from build123d import *

# Parameters (mm, degrees)
BOX_W           = 11
BOX_H           = 19
BOX_DEPTH       = 8
CHAMFER_SIZE    = 3
CHAMFER002_SIZE = 3


with BuildPart() as part:
    # Box → Box (new body)
    with BuildSketch(Plane.XY):
        with Locations((5.5, 9.5)):
            Rectangle(BOX_W, BOX_H)
    extrude(amount=BOX_DEPTH)

    # Chamfer
    chamfer_edges = [part.edges().sort_by_distance(p)[0] for p in [
        (11, 9.5, 8),
    ]]
    chamfer(chamfer_edges, length=CHAMFER_SIZE)

    # Chamfer002
    chamfer002_edges = [part.edges().sort_by_distance(p)[0] for p in [
        (0, 9.5, 8),
    ]]
    chamfer(chamfer002_edges, length=CHAMFER002_SIZE)


solid = part.part
Model file for the job. Use its own axes, mm. Round coordinates to 2 decimals unless told otherwise and drop trailing zeros. Order: outer loops, then holes, each group sorted by start corner. A loop starts at its lowest first (then second) coordinate and runs counter-clockwise, first axis right, second up.
(1) Band-saw the part on A-A (x = 2.25). List the corners of the cut face in (y, z), then the cut area to 3 significant figures.
(2) Band-saw the part on C-C (z = 6.5). List the corners of the cut face in (x, y).
(3) Drill centre lines: line 1 (Z direction, x = 2.5, y = 17.25); line 2 (Z direction, x = 0.5, y = 14.5); line 3 (X direction, y = 4.75, z = 7). Where is each one in solid material? Low to high.
(4) Band-saw the part on B-B (y = 2). List the corners of the cut face in (x, z), then the cut area to 3 significant figures.
Verdict:
1. outline: (0, 0) - (19, 0) - (19, 7.25) - (0, 7.25) - close
1. area: 138 mm2
2. outline: (1.5, 0) - (9.5, 0) - (9.5, 19) - (1.5, 19) - close
3. line 1: z = 0 to 7.5
3. line 2: z = 0 to 5.5
3. line 3: x = 2 to 9
4. outline: (0, 0) - (11, 0) - (11, 5) - (8, 8) - (3, 8) - (0, 5) - close
4. area: 79.0 mm2
